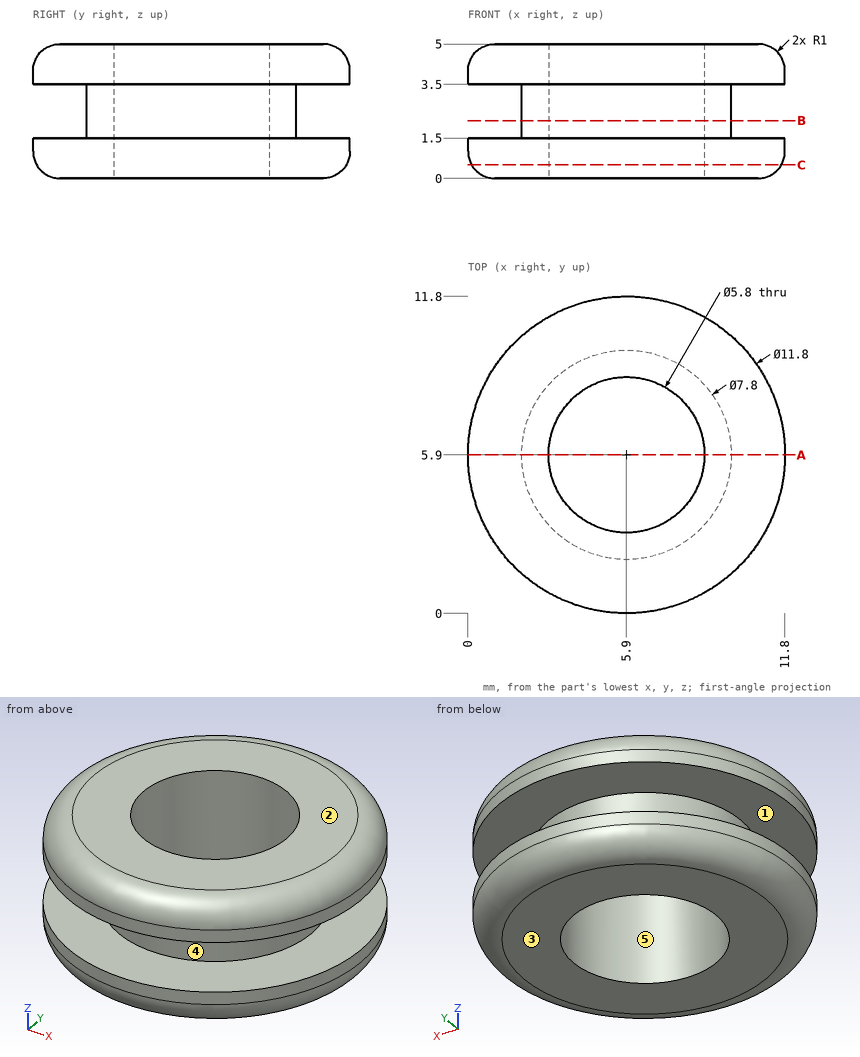
Study the drawing (mm; zero at the part's minimum x, y, z) and answer. A direction names the side the tool comes from. Give positions to 0.01 mm unless a question says otherwise; leave off trailing zeros. Write each loop counter-clockwise with the first axis right and the second up, starting at its lowest first coordinate (ties: lowest second). Pieces come first, ordered by that corner, then holes. Notation, with made-up numbers: (-33, -12.5) - (-15, -12.5) arc R7 ccw to (-15, -7.5) - close; hole circle Ø2 at (35, -30). An arc over 180 degrees is marked (long way). Use CSV: the item, a comma, the result in double quotes. Start each with the question number.
(1) Find section C-C (z = 0.5). Give the vertices of the cut face in (x, y).
(2) Determine the mould class of the marked faces 3, 4 and 5 for opening direction Z: +Z half, -Z half, draft (parallel to the pull), parting line (faces both ways), or undercut.
(3) Given P1, Ø1.5, axis at y = 3.5, z = 4, coming from the +X side; P2, Ø3, axis at y = 1.5, z = 2.5, coming from the +X side; P3, Ø2, axis at x = 6, y = 5, coming from the +Z side, each flat-ended and moving along its own axis, determine where each tip first touches the part or whether it passes through.
(4) Find section B-B (z = 2.15). Give the vertices of the cut face in (x, y), plus the area to 3 significant figures.
(5) For the marked faces 1 and 2, determine the directions among +Z, -Z, +X, -X, +Y, -Y from which every point of the face is accessible in a straight line to the end or side of a thin tool.
(6) Find section A-A (y = 5.9). Give the vertices of the cut face in (x, z).
(7) Consider line 1 along Y through (x, z) = (5.9, 2.1); line 2 along Y through (x, z) = (5.9, 1.25); line 3 along Z through (x, y) = (1.75, 7.75). Determine where each line is inside the solid, lowest interval first.
Findings below:
1,outline,"circle Ø11.53 at (5.9, 5.9); hole circle Ø5.8 at (5.9, 5.9)"
2,face 3,"-Z half"
2,face 4,"undercut"
2,face 5,"draft"
3,P1,"x = 11.56"
3,P2,"x = 10.8"
3,P3,"through"
4,outline,"circle Ø7.8 at (5.9, 5.9); hole circle Ø5.8 at (5.9, 5.9)"
4,area,"21.4 mm2"
5,face 1,"none"
5,face 2,"+Z, +X, -X, +Y, -Y"
6,outline,"(0, 1) arc R1 ccw to (1, 0) - (3, 0) - (3, 5) - (1, 5) arc R1 ccw to (0, 4) - (0, 3.5) - (2, 3.5) - (2, 1.5) - (0, 1.5) - close; (8.8, 0) - (10.8, 0) arc R1 ccw to (11.8, 1) - (11.8, 1.5) - (9.8, 1.5) - (9.8, 3.5) - (11.8, 3.5) - (11.8, 4) arc R1 ccw to (10.8, 5) - (8.8, 5) - close"
7,line 1,"2 to 3, 8.8 to 9.8"
7,line 2,"0 to 3, 8.8 to 11.8"
7,line 3,"0 to 1.5, 3.5 to 5"
